Autodesk Inventor part; units mm, degrees
ref_plane "YZ Plane" through (0, 0, 0) normal (1, 0, 0) x (0, 1, 0)
ref_plane "XZ Plane" through (0, 0, 0) normal (0, 1, 0) x (-1, 0, 0)
ref_plane "XY Plane" through (0, 0, 0) normal (0, 0, 1) x (1, 0, 0)
sketch "Sketch1" plane through (0, 0, 0) normal (0, 1, 0) x (-1, 0, 0)
  line L0 (55, 39) -> (55, -39)
  line L1 (55, -39) -> (-55, -39)
  line L2 (-55, -39) -> (-55, 39)
  line L3 (-55, 39) -> (55, 39)
  point P0 (0, 0)
  dimension "d0" = 78
  dimension "d1" = 110
  dimension "d2" = 55
  dimension "d3" = 39
extrude "Extrusion1" add sketch "Sketch1" along normal blind 10
sketch "Sketch2" plane through (0, 10, 0) normal (0, 1, 0) x (1, 0, 0)
  line L0 (-37.5, -39) -> (-37.5, -27)
  line L1 (-37.5, -27) -> (37.5, -27)
  line L2 (37.5, -27) -> (37.5, -39)
  line L3 (37.5, -39) -> (-37.5, -39)
  line L4 (-55, -39) -> (55, -39)
  point P0 (0, 0)
  point P1 (-37.5, -33)
  dimension "d6" = 12
  dimension "d8" = 37.5
  dimension "d9" = 75
  dimension "d14" = 33
extrude "Extrusion2" add sketch "Sketch2" along normal blind 35
sketch "Sketch3" plane through (-37.5, 45, 39) normal (0, 0, 1) x (1, 0, 0)
  circle A0 centre (17.5, -17.5) radius 6
  circle A1 centre (57.5, -17.5) radius 6
  line L0 (-17.5, -45) -> (92.5, -45)
  line L1 (0, 0) -> (75, 0)
  point P0 (37.5, -45)
  point P1 (37.5, 0)
  dimension "d16" = 12
  dimension "d17" = 12
  dimension "d18" = 27.5
  dimension "d19" = 27.5
  dimension "d20" = 40
  dimension "d21" = 20
extrude "Extrusion3" cut sketch "Sketch3" against normal blind 80
mirror "Mirror1" about plane through (0, 0, 0) normal (0, 0, 1) of "Extrusion2", "Extrusion3"
thread "Thread9"
thread "Thread13"
thread "Thread14"
thread "Thread15"
properties part number "Base Macaco" material "Steel AISI 4142 380 QT"
Could you check a few things on this model? Use its own coordinates, in mm. A direction names the side the tool comes from. Give positions to 0.01 mm unless a question says otherwise; leave off trailing zeros. Write each loop counter-clockwise with the first axis right and the second up, starting at its lowest first coordinate (ties: lowest second). Pieces come first, ordered by that corner, then holes. Notation, with made-up numbers: (22.25, 42) - (36.25, 42) arc R22 cw to (36.25, 73) - close; hole circle Ø7 at (-15.5, 75). An arc over 180 degrees is marked (long way). One line per item, written item: value. Start each with the question number.
Item 1: I'm going to push flat-ended pins straight in: pin 1 (6 mm diameter, centred on y = 24.5, z = -34, fed in from -X); pin 2 (1 mm diameter, centred on x = -38.5, z = 2.5, fed in from +Y); pin 3 (11 mm diameter, centred on x = 20, y = 27.5, fed in from +Z); pin 4 (9.5 mm diameter, centred on y = 33.5, z = 32, fed in from +X). Where does each tip first touch, or does it pass through?
Item 2: Imagine slicing it at A-A, the plane x = 20. List the corners of the cut face in (y, z) for me.
Item 3: Imagine slicing it at C-C, the plane y = 27.5. List the corners of the cut face in (x, z) for me, and give its area (3 significant figures).
Item 4: Please list where these lines run through material, in increasing order: line 1 (X direction, y = 27, z = -36); line 2 (Z direction, x = -11, y = 22.5); line 3 (Y direction, x = 20, z = 30.5). Write a range as from..to.
Item 5: If we mould it in two halves opening along Y, with no side actions, what happens to faces 5 (the face through (1, 0, 1)), 6 (the face through (-1, 45, 33)), 7 (the face through (-21.301, 21.643, 33.084))? For each: +Y half, -Y half, draft (parallel to the pull), parting line (faces both ways), or undercut.
Item 6: Which directions (+Z, -Z, +X, -X, +Y, -Y) give clear straight access to the entire face, cutting with the end or side of a thin tool? Please do faces 1 (the face through (-1, 27, 27)), 2 (the face through (37.5, 27, 33)), 3 (the face through (-37.5, 27, 33)), 4 (the face through (1, 22, 39)).
Item 7: Imagine slicing it at B-B, the plane y = 16.5. List the corners of the cut face in (x, z) for me.
Item 8: Imagine slicing it at D-D, the plane x = 34.5. List the corners of the cut face in (y, z) for me, and give its area (3 significant figures).
Geometry says:
1. pin 1: x = -37.5
1. pin 2: y = 10
1. pin 3: through
1. pin 4: x = 37.5
2. outline: (0, -39) - (21.5, -39) - (21.5, -27) - (10, -27) - (10, 27) - (21.5, 27) - (21.5, 39) - (0, 39) - close; (33.5, -39) - (45, -39) - (45, -27) - (33.5, -27) - close; (33.5, 27) - (45, 27) - (45, 39) - (33.5, 39) - close
3. outline: (-37.5, -39) - (-26, -39) - (-26, -27) - (-37.5, -27) - close; (-37.5, 27) - (-26, 27) - (-26, 39) - (-37.5, 39) - close; (-14, -39) - (14, -39) - (14, -27) - (-14, -27) - close; (-14, 27) - (14, 27) - (14, 39) - (-14, 39) - close; (26, -39) - (37.5, -39) - (37.5, -27) - (26, -27) - close; (26, 27) - (37.5, 27) - (37.5, 39) - (26, 39) - close
3. area: 1,220 mm^2
4. line 1: -37.5..-25.98, -14.02..14.02, 25.98..37.5
4. line 2: -39..-27, 27..39
4. line 3: 0..21.5, 33.5..45
5. face 5: -Y half
5. face 6: +Y half
5. face 7: undercut
6. face 1: +X, -X, +Y
6. face 2: +Z, -Z, +X, +Y
6. face 3: +Z, -Z, -X, +Y
6. face 4: +Z, +X, -X, +Y, -Y
7. outline: (-37.5, -39) - (37.5, -39) - (37.5, -27) - (-37.5, -27) - close; (-37.5, 27) - (37.5, 27) - (37.5, 39) - (-37.5, 39) - close
8. outline: (0, -39) - (45, -39) - (45, -27) - (10, -27) - (10, 27) - (45, 27) - (45, 39) - (0, 39) - close
8. area: 1,620 mm^2
